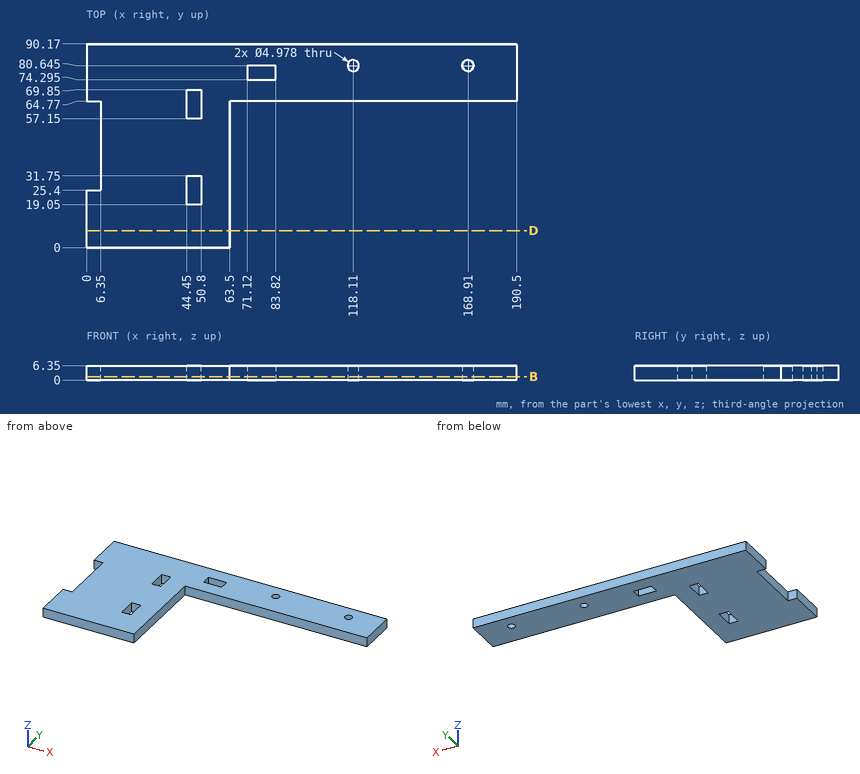
Design review of the part shown in the three views and the two pictorial views. Dimensions are in mm from the part's minimum x, y and z. Round coordinates to 2 decimals unless told otherwise and drop trailing zeros. Order: outer loops, then holes, each group sorted by start corner. A loop starts at its lowest first (then second) coordinate and runs counter-clockwise, first axis right, second up.
(1) Wall thickness on L1, parallel to Y at x = 168.91, z = 4.25 (1 decimal); L2, parallel to X at y = 60, z = 2.25; L3, parallel to Y at x = 81, z = 5.25 (1 decimal): over which ranges is each line inside the solid? List them lowest first.
Working result:
L1: y = 64.8 to 78.2, 83.1 to 90.2
L2: x = 6.35 to 44.45, 50.8 to 63.5
L3: y = 64.8 to 74.3, 80.6 to 90.2
(2) Take a section at D-D, the plane y = 7.5. State the section outline as (x, z) points, plus the area to 3 significant figures.
Working result:
outline: (0, 0) - (63.5, 0) - (63.5, 6.35) - (0, 6.35) - close
area: 403 mm2
(3) For P1, Ø2, axis at x = 133, z = 3, coming from the -Y side; P2, Ø3, axis at y = 23.5, z = 2, coming from the +X side, all flat-tipped, find the tip position at first contact; note any pin that passes through.
Working result:
P1: stops at y = 64.77
P2: stops at x = 63.5
(4) Take a section at B-B, the plane z = 1.5. Count the separate pieces of the cut face and the enclosed holes in it, plus the area to 3 significant figures.
Working result:
separate pieces: 1
enclosed holes: 5
area: 8,420 mm2
